Geometry check sheet. Reference: drawing and pictorial views, mm from the part's lowest x, y, z. A direction names the side the tool comes from. Give positions to 0.01 mm unless a question says otherwise; leave off trailing zeros. Loops run counter-clockwise (first coordinate to the right, second up) from the corner with the lowest first, then second, coordinate; pieces in that order, holes last. Notation, with made-up numbers: (-36, 87.25) - (9, 87.25) arc R8 cw to (9, 91.25) - close; hole circle Ø7 at (10, 65.5). An arc over 180 degrees is marked (long way). Answer in a Markdown table with one row per item. Add a question column.
(1) Sectioned sample at D-D on y = 2.5. Enter the section's corners in (x, z) (1 decimal).
(2) Sectioned sample at C-C on y = 6. Enter the section's corners in (x, z) (1 decimal).
(3) Thickness scan on L1, parallel to Z at x = 5.5, y = 6.5; L2, parallel to Z at x = 2.5, y = 7.75; L3, parallel to X at y = 6.25, z = 6.5. Record the ranges inside material, lowest first.
(4) Draft check along Y on the marked faces 4, 5 and 6. Enter one of: released by +Y, released by -Y, zero draft, split by the parting line, or undercut.
(5) Go/stop test with flat-tipped pins: P1, Ø2.5, axis at x = 5, z = 0.5, coming from the +Y side; P2, Ø2, axis at x = 7.5, z = 5.5, coming from the -Y side; P3, Ø4, axis at x = 9.5, z = 20.5, coming from the -Y side (1 decimal). Record where each tip stops, or that it passes through.
(6) Sectioned sample at A-A on x = 5.25. Enter the section's corners in (y, z), then the cut area to 3 significant figures.
(7) Sectioned sample at B-B on z = 6.25. Enter the section's corners in (x, y), then the cut area to 3 significant figures.
(8) Set-up check for the marked faces 1, 2 and 3: record each of +Z, -Z, +X, -X, +Y, -Y from which the full face is reachable in a straight line by a thin tool's end or side.
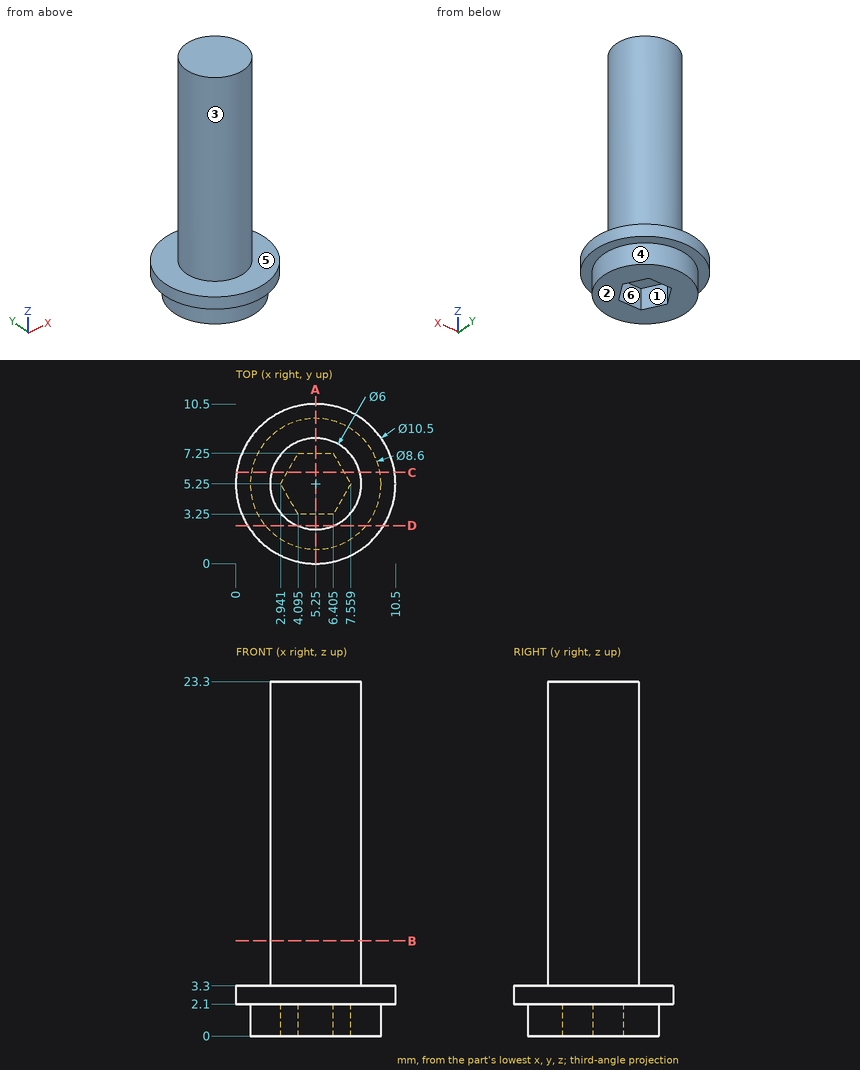
Reply:
| question | item | result |
|---|---|---|
| 1 | outline | (0.8, 2.1) - (1.9, 2.1) - (1.9, 0) - (8.6, 0) - (8.6, 2.1) - (9.7, 2.1) - (9.7, 3.3) - (6.4, 3.3) - (6.4, 23.3) - (4.1, 23.3) - (4.1, 3.3) - (0.8, 3.3) - close |
| 2 | outline | (0.1, 2.1) - (1, 2.1) - (1, 0) - (3.4, 0) - (3.4, 2.1) - (7.1, 2.1) - (7.1, 0) - (9.5, 0) - (9.5, 2.1) - (10.4, 2.1) - (10.4, 3.3) - (8.2, 3.3) - (8.2, 23.3) - (2.3, 23.3) - (2.3, 3.3) - (0.1, 3.3) - close |
| 3 | L1 | 2.1 to 23.3 |
| 3 | L2 | 0 to 3.3 |
| 3 | L3 | 2.42 to 8.08 |
| 4 | face 4 | split by the parting line |
| 4 | face 5 | zero draft |
| 4 | face 6 | undercut |
| 5 | P1 | y = 9.55 |
| 5 | P2 | y = 2.52 |
| 5 | P3 | y = 3.3 |
| 6 | outline | (0, 2.1) - (0.95, 2.1) - (0.95, 0) - (3.25, 0) - (3.25, 2.1) - (7.25, 2.1) - (7.25, 0) - (9.55, 0) - (9.55, 2.1) - (10.5, 2.1) - (10.5, 3.3) - (8.25, 3.3) - (8.25, 23.3) - (2.25, 23.3) - (2.25, 3.3) - (0, 3.3) - close |
| 6 | area | 142 mm^2 |
| 7 | outline | circle Ø6 at (5.25, 5.25) |
| 7 | area | 28.3 mm^2 |
| 8 | face 1 | -Z |
| 8 | face 2 | -Z, +X, -X, +Y, -Y |
| 8 | face 3 | +Z |
